Part model, mm, in its own coordinate system. A direction names the side the tool comes from. Coordinates: 2 decimals unless noted, no trailing zeros. Order: outer loops, then holes, each group sorted by start corner. A loop starts at its lowest first (then second) coordinate and runs counter-clockwise, first axis right, second up.
```python
from build123d import *

# Parameters (mm, degrees)
F0_W            = 8
F0_H            = 17.5
F3_D            = 6
F4_T            = -2
F6_D            = 8
F6_COPIES_COUNT = 5
F7_SIZE         = 1


# Not quite as in the source:
# - a pattern or mirror of a feature is missing from the dataset's text; its kind, count and spacing are read off the source's solid


with BuildPart() as f1:
    # F0 (on Top) → F1 (revolve)
    with BuildSketch(Plane.XY):
        with Locations((4, 8.75)):
            Rectangle(F0_W, F0_H)
    revolve(axis=Axis((4, 0, 0), (1, 0, 0)))

    # F3 (through all)
    with Locations(Plane(origin=(0, 0, 0), x_dir=(0, 1, 0), z_dir=(-1, 0, 0))):
        with Locations((0, 0)):
            Hole(F3_D / 2)

    # F4
    f4_openings = [f1.faces().sort_by_distance(p)[0] for p in [
        (8, -17.005025, 0),
    ]]
    offset(amount=F4_T, openings=f4_openings)

    # F6 (through all)
    with Locations(Plane(origin=(0, 0, 0), x_dir=(0, 1, 0), z_dir=(-1, 0, 0))):
        with Locations((0, -10)):
            f6 = Hole(F6_D / 2)

    # F6_copies: F6 ×5 about axis
    f6_copies_axis = Axis((0, 0, 0), (1, 0, 0))
    for i in range(1, F6_COPIES_COUNT):
        add(f6.rotate(f6_copies_axis, i * 360 / F6_COPIES_COUNT), mode=Mode.SUBTRACT)

    # F7
    f7_edges = [f1.edges().sort_by_distance(p)[0] for p in [
        (8, -5, 0),
    ]]
    chamfer(f7_edges, length=F7_SIZE)


solid = f1.part
```
(1) Drop flat-ended pins along their axis: pin 1 (7 mm diameter, centred on y = 5.88, z = -8.09, fed in from -X); pin 2 (2 mm diameter, centred on x = 5, y = -6, fed in from -Z); pin 3 (1.5 mm diameter, centred on x = 6, y = -13, fed in from -Z); pin 4 (1.5 mm diameter, centred on x = 2.5, y = -5.5, fed in from +Z). Give the stop position or say it passes through.
(2) Slice it at B-B, the plane z = -8.5. Give the cut face in (x, y).
(3) Slice it at D-D, the plane z = 10. Give the cut face in (x, y).
(4) Probe line 1 (Z direction, x = 1.1, y = 0); line 2 (Z direction, x = 3.75, y = 0); line 3 (Z direction, x = 7.5, y = 0.5). List the from-to ranges inside material, lowest first.
(5) Tool access for faces 1 (the face through (5.042, -2.018, 15.368)), 2 (the face through (1.014, 0.867, 13.905)): list every direction of +Z, -Z, +X, -X, +Y, -Y with a clear straight run to the whole face (end or side of a thin tool).
(6) Slice it at C-C, the plane x = 4.75. Give the cut face in (y, z).
(7) Slice it at A-A, the plane y = 0. Give the cut face in (x, z).
Here are the results:
1. pin 1: passes through
1. pin 2: stops at z = -16.77
1. pin 3: stops at z = -12.5
1. pin 4: stops at z = 16.84
2. outline: (0, -15.3) - (8, -15.3) - (8, -12.96) - (2, -12.96) - (2, -9.86) - (0, -9.86) - close; (0, -1.9) - (2, -1.9) - (2, 1.9) - (0, 1.9) - close; (0, 9.86) - (2, 9.86) - (2, 12.96) - (8, 12.96) - (8, 15.3) - (0, 15.3) - close
3. outline: (0, -14.36) - (8, -14.36) - (8, -11.84) - (2, -11.84) - (2, -4) - (0, -4) - close; (0, 4) - (2, 4) - (2, 11.84) - (8, 11.84) - (8, 14.36) - (0, 14.36) - close
4. line 1: z = -17.5 to -3, 3 to 6, 14 to 17.5
4. line 2: z = -17.5 to -15.5, -5 to -3, 3 to 5, 15.5 to 17.5
4. line 3: z = -17.49 to -15.49, -4.47 to -2.96, 2.96 to 4.47, 15.49 to 17.49
5. face 1: +X
5. face 2: +X, -X
6. outline: circle Ø35 at (0, 0); circle Ø10 at (0, 0); hole circle Ø31 at (0, 0); hole circle Ø6 at (0, 0)
7. outline: (0, -17.5) - (8, -17.5) - (8, -15.5) - (2, -15.5) - (2, -5) - (7, -5) - (8, -4) - (8, -3) - (0, -3) - close; (0, 3) - (8, 3) - (8, 4) - (7, 5) - (2, 5) - (2, 6) - (0, 6) - close; (0, 14) - (2, 14) - (2, 15.5) - (8, 15.5) - (8, 17.5) - (0, 17.5) - close
